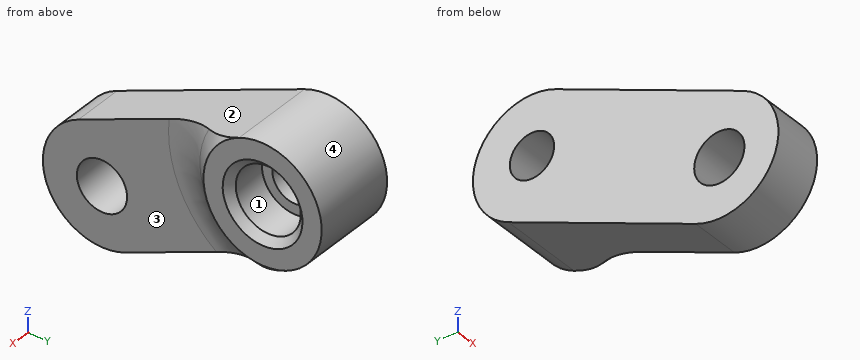
```python
from build123d import *

# Parameters (mm, degrees)
BOSS_EXTRUDE1_DEPTH = 5.75
CUT_EXTRUDE1_DEPTH  = 2.35
HOLE1_D             = 3.4
HOLE2_D             = 3
HOLE2_CBORE_D       = 4.4
HOLE2_CBORE_DEPTH   = 2.8
CHAMFER1_SIZE       = 0.5
FILLET1_R           = 4.4


# Read off the part's stored shape, not the designer's step: Draft1
with BuildPart() as part:
    # Sketch1 → Boss-Extrude1 (new body)
    with BuildSketch(Plane(origin=(-31.596370889, 0, 0), x_dir=(0, 0, -1), z_dir=(1, 0, 0))):
        with BuildLine():
            Line((30.830485373, -54.332845156), (36.330485373, -67.009692228))
            ThreePointArc((36.330485373, -67.009692228), (41.592062311, -69.087144543), (43.669514627, -63.825567605))
            Line((43.669514627, -63.825567605), (38.169514627, -51.148720534))
            ThreePointArc((38.169514627, -51.148720534), (32.907937689, -49.071268218), (30.830485373, -54.332845156))
        make_face()
    extrude(amount=-BOSS_EXTRUDE1_DEPTH)

    # Sketch2 → Cut-Extrude1 (cut)
    with BuildSketch(Plane(origin=(-31.596370889, 0, 0), x_dir=(0, 0, -1), z_dir=(1, 0, 0))):
        with BuildLine():
            Line((32.793412497, -58.857159149), (36.330485373, -67.009692228))
            ThreePointArc((36.330485373, -67.009692228), (41.592062311, -69.087144543), (43.669514627, -63.825567605))
            Line((43.669514627, -63.825567605), (40.132441751, -55.673034527))
            ThreePointArc((40.132441751, -55.673034527), (37.027398919, -58.566137315), (32.793412497, -58.857159149))
        make_face()
    extrude(amount=-CUT_EXTRUDE1_DEPTH, mode=Mode.SUBTRACT)

    # Draft1 outline → Draft1 (revolve, cut)
    with BuildSketch(Plane(origin=(0, -52.740782845, -34.5), x_dir=(0, 1, 0), z_dir=(0, 0, -1))):
        Polygon((6.35, -31.596367589), (3.9999967, -31.596367589), (6.35, -33.946370889), align=None)
    revolve(axis=Axis((0, -52.740782845, -34.5), (1, 0, 0)), mode=Mode.SUBTRACT)

    # Hole1 (through all)
    with Locations(Plane.ZY.offset(37.346370889)):
        with Locations((-40, -65.417629916)):
            Hole(HOLE1_D / 2)

    # Hole2 (through all)
    with Locations(Plane(origin=(-31.596370889, 0, 0), x_dir=(0, 0, -1), z_dir=(1, 0, 0))):
        with Locations((34.5, -52.740782845)):
            CounterBoreHole(HOLE2_D / 2, HOLE2_CBORE_D / 2, HOLE2_CBORE_DEPTH)

    # Chamfer1
    chamfer1_edges = [part.edges().sort_by_distance(p)[0] for p in [
        (-31.596370889, -52.740782845, -32.3),
    ]]
    chamfer(chamfer1_edges, length=CHAMFER1_SIZE)

    # Fillet1
    fillet1_edges = [part.edges().sort_by_distance(p)[0] for p in [
        (-33.946370889, -58.566137315, -37.027398919),
    ]]
    fillet(fillet1_edges, radius=FILLET1_R)


solid = part.part
```
Geometry: final body of the model. Coordinates: model frame, mm. Face numbers are marked on the shaded views. Coordinates: 2 decimals unless noted, no trailing zeros. Order: outer loops, then holes, each group sorted by start corner. A loop starts at its lowest first (then second) coordinate and runs counter-clockwise, first axis right, second up. Notation, with made-up numbers: (30.25, 59) - (58.25, 59) arc R21 cw to (58.25, 84) - close; hole circle Ø2 at (10.25, -4). An arc over 180 degrees is marked (long way). Return JSON: item names as keys, results as strings. Group by question number.
1. Cut plane A-A (y = -65). Output: boundary loops of the cut face in (x, z), plus the area to 3 significant figures.
2. Pin query (flat end, axial travel): pin 1 (2.5 mm diameter, centred on y = -52.74, z = -34.5, fed in from +X); pin 2 (3 mm diameter, centred on x = -35, y = -52, fed in from -Z); pin 3 (1 mm diameter, centred on x = -32.5, z = -32.5, fed in from +Y); pin 4 (5 mm diameter, centred on y = -57, z = -40, fed in from +X). Return the tip coordinate at first contact, or that it passes through.
3. Material intervals for line 1 along X through (y, z) = (-63.75, -35); line 2 along X through (y, z) = (-51.75, -32.5); line 3 along Z through (x, y) = (-34.1, -54.5), sorted ascending. Write a range as [from, to].
4. Pull-direction query (Y, two-part tool) for the marked faces 1, 2, 3 and 4; classes: pulls with the +Y half, pulls with the -Y half, needs draft (parallel to the pull), parting line crosses it, or undercut.
5. Cut plane B-B (x = -34.6). Output: boundary loops of the cut face in (y, z), plus the area to 3 significant figures.
6. Cut plane D-D (x = -33.25). Output: boundary loops of the cut face in (y, z).
7. Cut plane C-C (z = -34.5). Output: boundary loops of the cut face in (x, y), plus the area to 3 significant figures.
Resolved:
{
 "1": {"outline": "(-37.35, -43.98) - (-33.95, -43.98) - (-33.95, -41.65) - (-37.35, -41.65) - close; (-37.35, -38.35) - (-33.95, -38.35) - (-33.95, -35.46) - (-37.35, -35.46) - close", "area": "17.8 mm²"},
 "2": {"pin 1": "passes through", "pin 2": "stops at z = -39.19", "pin 3": "stops at y = -49.03", "pin 4": "stops at x = -32.05"},
 "3": {"line 1": "x = [-37.35, -33.95]", "line 2": "x = [-37.35, -32.06]", "line 3": "z = [-39.62, -35.82], [-33.18, -30.9]"},
 "4": {"face 1": "undercut", "face 2": "pulls with the -Y half", "face 3": "needs draft", "face 4": "parting line crosses it"},
 "5": {"outline": "(-67.01, -36.33) arc R4 ccw to (-63.83, -43.67) - (-51.15, -38.17) arc R4 ccw to (-54.33, -30.83) - close; hole circle Ø3.4 at (-65.42, -40); hole circle Ø3 at (-52.74, -34.5)", "area": "145 mm²"},
 "6": {"outline": "(-58.18, -32.5) arc R5.8 ccw to (-55, -39.84) - (-51.15, -38.17) arc R4 ccw to (-54.33, -30.83) - close; hole circle Ø4.4 at (-52.74, -34.5)"},
 "7": {"outline": "(-37.35, -62.79) - (-33.95, -62.79) - (-33.95, -60.91) arc R4.4 cw to (-32.66, -57.8) - (-31.6, -56.74) - (-31.6, -55.44) - (-32.1, -54.94) - (-34.4, -54.94) - (-34.4, -54.24) - (-37.35, -54.24) - close; (-37.35, -51.24) - (-34.4, -51.24) - (-34.4, -50.54) - (-32.1, -50.54) - (-31.6, -50.04) - (-31.6, -48.74) - (-37.35, -48.74) - close", "area": "48.3 mm²"}
}
